Can you work these out from the drawing? Everything is in mm from the part's minimum corner. A direction names the side the tool comes from. Round coordinates to 2 decimals unless told otherwise and drop trailing zeros. Loops run counter-clockwise (first coordinate to the right, second up) from the corner with the lowest first, then second, coordinate; pieces in that order, holes last. Notation, with made-up numbers: M 9,13 L 56,13 A26 ccw 56,34 Z; hole C 89.5,15.5 d2. An arc over 180 degrees is marked long. Use a Markdown table: item, result.
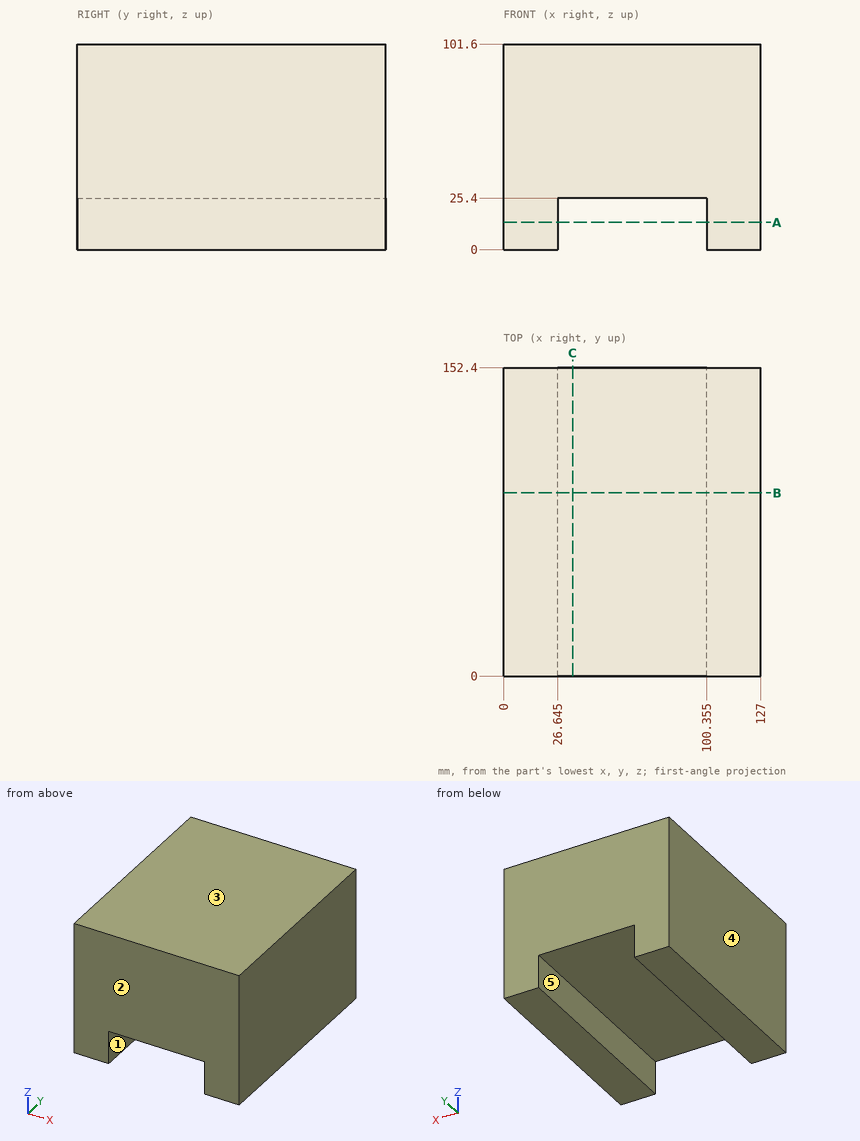
Q1. Imagine slicing it at A-A, the plane z = 13.5. Please give me the cut outline in (x, y) (1 decimal), then the cut area to 3 significant figures.
Return value:
| item | result |
|---|---|
| outline | M 0,0 L 26.6,0 L 26.6,152.4 L 0,152.4 Z; M 100.4,0 L 127,0 L 127,152.4 L 100.4,152.4 Z |
| area | 8,120 mm^2 |
Q2. Imagine slicing it at C-C, the plane x = 34. Please give me the cut outline in (y, z), then the cut area to 3 significant figures.
Return value:
| item | result |
|---|---|
| outline | M 0,25.4 L 152.4,25.4 L 152.4,101.6 L 0,101.6 Z |
| area | 11,600 mm^2 |
Q3. I need wall thicknesses on line 1 (Z direction, x = 86, y = 36.5); line 2 (X direction, y = 60, z = 13) (1 decimal). Which ranges of each line are inside material? Lowest first, please. Write a range as from..to.
Return value:
| item | result |
|---|---|
| line 1 | z = 25.4..101.6 |
| line 2 | x = 0..26.6, 100.4..127 |
Q4. For the marked faces 1 and 2, which set-ups out of +Z, -Z, +X, -X, +Y, -Y let a thin tool reach every point of the face, with its end or its side?
Return value:
| item | result |
|---|---|
| face 1 | -Z, +Y, -Y |
| face 2 | +Z, -Z, +X, -X, -Y |
Q5. Imagine slicing it at B-B, the plane y = 90.5. Please give me the cut outline in (x, z) (1 decimal), then the cut area to 3 significant figures.
Return value:
| item | result |
|---|---|
| outline | M 0,0 L 26.6,0 L 26.6,25.4 L 100.4,25.4 L 100.4,0 L 127,0 L 127,101.6 L 0,101.6 Z |
| area | 11,000 mm^2 |
Q6. We'd pull the mould along X, two halves only. Please class the marked faces 3, 4 and 5: pulls with the +X half, pulls with the -X half, needs draft (parallel to the pull), parting line crosses it, or undercut.
Return value:
| item | result |
|---|---|
| face 3 | needs draft |
| face 4 | pulls with the -X half |
| face 5 | undercut |
